```python
from build123d import *

# Parameters (mm, degrees)
BOSS_EXTRUDE1_DEPTH = 7.9375
FILLET2_R           = 12.7
CHAMFER1_SIZE       = 8.198155848
CHAMFER1_SIZE_2     = 7.9375


with BuildPart() as part:
    # Sketch1 → Boss-Extrude1 (new body)
    with BuildSketch(Plane(origin=(0, 0, 0), x_dir=(1, 0, 0), z_dir=(0, 1, 0))):
        with BuildLine():
            Line((-7.9502, 133.6675), (7.9502, 133.6675))
            Line((7.9502, 133.6675), (7.9502, 59.79882896))
            ThreePointArc((7.9502, 59.79882896), (42.656216575, 42.656216575), (59.79882896, 7.9502))
            Line((59.79882896, 7.9502), (133.6675, 7.9502))
            Line((133.6675, 7.9502), (133.6675, -7.9502))
            Line((133.6675, -7.9502), (59.79882896, -7.9502))
            ThreePointArc((59.79882896, -7.9502), (42.656216575, -42.656216575), (7.9502, -59.79882896))
            Line((7.9502, -59.79882896), (7.9502, -133.6675))
            Line((7.9502, -133.6675), (-7.9502, -133.6675))
            Line((-7.9502, -133.6675), (-7.9502, -59.79882896))
            ThreePointArc((-7.9502, -59.79882896), (-42.656216575, -42.656216575), (-59.79882896, -7.9502))
            Line((-59.79882896, -7.9502), (-133.6675, -7.9502))
            Line((-133.6675, -7.9502), (-133.6675, 7.9502))
            Line((-133.6675, 7.9502), (-59.79882896, 7.9502))
            ThreePointArc((-59.79882896, 7.9502), (-42.656216575, 42.656216575), (-7.9502, 59.79882896))
            Line((-7.9502, 59.79882896), (-7.9502, 133.6675))
        make_face()
        with BuildLine():
            Line((-1.6002, 51.092447252), (-1.6002, 127.3175))
            Line((-1.6002, 127.3175), (1.6002, 127.3175))
            Line((1.6002, 127.3175), (1.6002, 51.092447252))
            ThreePointArc((1.6002, 51.092447252), (36.145530887, 36.145530887), (51.092447252, 1.6002))
            Line((51.092447252, 1.6002), (127.3175, 1.6002))
            Line((127.3175, 1.6002), (127.3175, -1.6002))
            Line((127.3175, -1.6002), (51.092447252, -1.6002))
            ThreePointArc((51.092447252, -1.6002), (36.145530887, -36.145530887), (1.6002, -51.092447252))
            Line((1.6002, -51.092447252), (1.6002, -127.3175))
            Line((1.6002, -127.3175), (-1.6002, -127.3175))
            Line((-1.6002, -127.3175), (-1.6002, -51.092447252))
            ThreePointArc((-1.6002, -51.092447252), (-36.145530887, -36.145530887), (-51.092447252, -1.6002))
            Line((-51.092447252, -1.6002), (-127.3175, -1.6002))
            Line((-127.3175, -1.6002), (-127.3175, 1.6002))
            Line((-127.3175, 1.6002), (-51.092447252, 1.6002))
            ThreePointArc((-51.092447252, 1.6002), (-36.145530887, 36.145530887), (-1.6002, 51.092447252))
        make_face(mode=Mode.SUBTRACT)
    extrude(amount=BOSS_EXTRUDE1_DEPTH)

    # Fillet2
    fillet2_edges = [part.edges().sort_by_distance(p)[0] for p in [
        (59.79882896, 3.96875, 7.9502),
        (7.9502, 3.96875, 59.79882896),
        (-7.9502, 3.96875, 59.79882896),
        (-59.79882896, 3.96875, 7.9502),
        (-59.79882896, 3.96875, -7.9502),
        (-7.9502, 3.96875, -59.79882896),
        (7.9502, 3.96875, -59.79882896),
        (59.79882896, 3.96875, -7.9502),
    ]]
    fillet(fillet2_edges, radius=FILLET2_R)

    # Chamfer1
    # the kernel refuses this chamfer: 8.198155848, 7.9375 mm, written as the material it takes off along each edge
    with BuildSketch(Plane(origin=(-1.6002, -22.411946767, -51.092447252), x_dir=(-0.9932071944131365, 0, 0.11635922381137723), z_dir=(0, 1, 0))) as chamfer1_piece_1:
        with BuildLine():
            Line((8.711494705, 0), (-CHAMFER1_SIZE * 0.116359223814, -CHAMFER1_SIZE * 0.993207194436))
            Line((-CHAMFER1_SIZE * 0.116359223814, -CHAMFER1_SIZE * 0.993207194436), (0, 0))
            ThreePointArc((0, 0), (4.4818633, -0.185760204), (8.711494705, 0))
        make_face()
    extrude(amount=52.761393535, mode=Mode.SUBTRACT)
    with BuildSketch(Plane(origin=(-51.092447252, -23.390114348, -1.6002), x_dir=(0.12010619986132272, 0, -0.9927610491728973), z_dir=(0, 1, 0)), Plane(origin=(-1.6002, -23.390114348, 51.092447252), x_dir=(-0.9927610491728978, 0, -0.12010619986131951), z_dir=(0, 1, 0)), Plane(origin=(51.092447252, -23.390114348, 1.6002), x_dir=(-0.12010619986131572, 0, 0.9927610491728983), z_dir=(0, 1, 0)), Plane(origin=(1.6002, -23.390114348, -51.092447252), x_dir=(0.9927610491728988, 0, 0.12010619986131156), z_dir=(0, 1, 0))) as chamfer1_piece_2:
        with BuildLine():
            Line((9.0958069, 0), (-CHAMFER1_SIZE_2 * 0.120106199861, CHAMFER1_SIZE_2 * 0.992761049173))
            Line((-CHAMFER1_SIZE_2 * 0.120106199861, CHAMFER1_SIZE_2 * 0.992761049173), (0, 0))
            ThreePointArc((0, 0), (4.677699861, 0.202549732), (9.0958069, 0))
        make_face()
    extrude(amount=54.717728697, mode=Mode.SUBTRACT)
    with BuildSketch(Plane(origin=(-51.092447252, -22.411946767, 1.6002), x_dir=(-1, 0, 0), z_dir=(0, 1, 0)), Plane(origin=(1.6002, -22.411946767, 51.092447252), x_dir=(0, 0, 1), z_dir=(0, 1, 0)), Plane(origin=(51.092447252, -22.411946767, -1.6002), x_dir=(1, 0, 0), z_dir=(0, 1, 0))) as chamfer1_piece_3:
        with BuildLine():
            Line((CHAMFER1_SIZE, 0), (-1.013662762, 8.652319215))
            ThreePointArc((-1.013662762, 8.652319215), (-0.337007764, 4.473033787), (0, 0))
            Line((0, 0), (CHAMFER1_SIZE, 0))
        make_face()
    extrude(amount=52.761393535, mode=Mode.SUBTRACT)


solid = part.part
```
The listing builds one solid part. Answer for the finished solid, in the listing's coordinates (mm). A direction names the side the tool comes from. Give positions to 0.01 mm unless a question says otherwise; leave off trailing zeros. Order: outer loops, then holes, each group sorted by start corner. A loop starts at its lowest first (then second) coordinate and runs counter-clockwise, first axis right, second up. Notation, with made-up numbers: (-29, 61.5) - (-1, 61.5) arc R16 ccw to (-1, 65.5) - close; hole circle Ø9 at (43, 19). An arc over 180 degrees is marked (long way). Use one line per item in the form item = value. Start each with the question number.
(1) The mould has two halves that part along Z. Classify faces 1 (the cylindrical face through (-36.3, 3.91, -35.99)), 2 (the flat face through (-101, 4, 7.95)), 3 (the flat face through (20, 0, -50)): released by +Z, released by -Z, zero draft, split by the parting line, or undercut.
(2) A cutting plane is placed at A-A, the plane x = -76.5. Write down the section's boundary in (y, z).
(3) Flat-ended cylindrical pins translate along their axes: pin 1 Ø4 at (x, y) = (95.5, 5) entering from +Z; pin 2 Ø2.5 at (y, z) = (3, -87.5) entering from -X; pin 3 Ø4 at (x, y) = (-17, 2.5) entering from +Z; pin 4 Ø1 at (x, z) = (34, 41.5) entering from -Y. Find the tip coordinate at first contact, or state that the pin passes through.
(4) Consider line 1 (Z direction, x = 109, y = 1.75); line 2 (Z direction, x = -1, y = 6). Determine where each line is inside the solid, lowest interval first. Write a range as from..to.
(5) A cutting plane is placed at B-B, the plane z = 79. Write down the section's boundary in (x, y), then the cut area to 3 significant figures.
(6) For faces 4 (the flat face through (102, 4, 7.95)), 5 (the flat face through (-102, 4, -7.95)), 6 (the flat face through (-94, 4, -1.6)), 7 (the cylindrical face through (-42.36, 3.91, 42.95)), 8 (the flat face through (7.95, 4, -102)), determine the directions among +Z, -Z, +X, -X, +Y, -Y from which every point of the face is accessible in a straight line to the end or side of a thin tool.
Ans:
q1.face_1 = undercut
q1.face_2 = released by +Z
q1.face_3 = zero draft
q2.outline = (0, -7.95) - (7.94, -7.95) - (7.94, -1.6) - (0, -1.6) - close; (0, 1.6) - (7.94, 1.6) - (7.94, 7.95) - (0, 7.95) - close
q3.pin_1 = 7.95
q3.pin_2 = -7.95
q3.pin_3 = 58.67
q3.pin_4 = 0
q4.line_1 = -7.95..-1.6, 1.6..7.95
q4.line_2 = -133.67..-127.32, 127.32..133.67
q5.outline = (-7.95, 0) - (-1.6, 0) - (-1.6, 7.94) - (-7.95, 7.94) - close; (1.6, 0) - (7.95, 0) - (7.95, 7.94) - (1.6, 7.94) - close
q5.area = 101 mm^2
q6.face_4 = +Z, +X, +Y, -Y
q6.face_5 = -Z, -X, +Y, -Y
q6.face_6 = +Y, -Y
q6.face_7 = +Z, -X, +Y, -Y
q6.face_8 = -Z, +X, +Y, -Y
